Source: CAD feature listing. Evaluate the final solid. Frame: model axes, mm. Round coordinates to 2 decimals unless told otherwise and drop trailing zeros. Write each loop counter-clockwise with the first axis right and the second up, starting at its lowest first coordinate (ties: lowest second). Pieces come first, ordered by that corner, then holes. Notation, with made-up numbers: (-3.75, -35.5) -> (46.25, -35.5) arc R18 ccw to (46.25, -14.5) -> close; hole circle Ø6 at (51, -26). An arc over 180 degrees is marked (long way). Return JSON: item names as keys, results as strings. Group by question number.
from build123d import *

# Parameters (mm, degrees)
AUFSATZ_LINEAR_START            = 3
SKIZZE2_R                       = 3
AUFSATZ_LINEAR_AUSTRAGEN1_DEPTH = 6


with BuildPart() as part:
    # Skizze2 → Aufsatz-Linear austragen1 (new body)
    with BuildSketch(Plane.XY.offset(AUFSATZ_LINEAR_START)):
        with BuildLine():
            Line((0, 675), (70, 675))
            ThreePointArc((70, 675), (75, 670), (70, 665))
            Line((70, 665), (0, 665))
            ThreePointArc((0, 665), (-5, 670), (0, 675))
        make_face()
        with Locations((0, 670)):
            Circle(SKIZZE2_R, mode=Mode.SUBTRACT)
        with Locations((70, 670)):
            Circle(SKIZZE2_R, mode=Mode.SUBTRACT)
    extrude(amount=AUFSATZ_LINEAR_AUSTRAGEN1_DEPTH)


solid = part.part
Item 1: Cut plane A-A on y = 670. Output: boundary loops of the cut face in (x, z).
Item 2: Cut plane C-C on y = 666. Output: boundary loops of the cut face in (x, z), and give its area (3 significant figures).
Item 3: Cut plane D-D on y = 674.25. Output: boundary loops of the cut face in (x, z), and give its area (3 significant figures).
Item 4: Cut plane B-B on z = 4.55. Output: boundary loops of the cut face in (x, y).
Item 5: Material intervals for probe 1 along X at (y, z) = (670, 5.25); probe 2 along Y at (x, z) = (0, 7.85); probe 3 along X at (y, z) = (672, 5.2), sorted ascending.
Here are the results:
{
 "1": {"outline": "(-5, 3) -> (-3, 3) -> (-3, 9) -> (-5, 9) -> close; (3, 3) -> (67, 3) -> (67, 9) -> (3, 9) -> close; (73, 3) -> (75, 3) -> (75, 9) -> (73, 9) -> close"},
 "2": {"outline": "(-3, 3) -> (73, 3) -> (73, 9) -> (-3, 9) -> close", "area": "456 mm^2"},
 "3": {"outline": "(-2.63, 3) -> (72.63, 3) -> (72.63, 9) -> (-2.63, 9) -> close", "area": "452 mm^2"},
 "4": {"outline": "(0, 665) -> (70, 665) arc R5 ccw to (70, 675) -> (0, 675) arc R5 ccw to start; hole circle Ø6 at (0, 670); hole circle Ø6 at (70, 670)"},
 "5": {"probe 1": "x = -5 to -3, 3 to 67, 73 to 75", "probe 2": "y = 665 to 667, 673 to 675", "probe 3": "x = -4.58 to -2.24, 2.24 to 67.76, 72.24 to 74.58"}
}
